For this review, take the finished solid that the model builds, in its own axes (mm). Coordinates: 2 decimals unless noted, no trailing zeros. Loops run counter-clockwise (first coordinate to the right, second up) from the corner with the lowest first, then second, coordinate; pieces in that order, holes last. Notation, with made-up numbers: (-30.75, 51) - (-21.75, 51) arc R32 cw to (-21.75, 77) - close; hole circle Ø7 at (51, 20). An arc over 180 degrees is marked (long way). One line per item, written item: value. Start each with the question number.
1. Take a section at B-B, the plane x = -1.7. State the section outline as (y, z) points.
2. To check wall thickness, follow line 1 (Z direction, x = -0.35, y = 0); line 2 (Z direction, x = 0.35, y = 3.75); line 3 (Y direction, x = -0.55, z = 1.5). State the ranges of each line that lie inside material, in increasing order. Write a range as from..to.
3. The part is to be moulded in two halves that separate along Y. For faces 1 (the face through (0, 0, -7)), 2 (the face through (1.893, -7.184, -0.158)), 3 (the face through (0.02, -3.54, -2.71)), say which applies: released by +Y, released by -Y, zero draft, split by the parting line, or undercut.
4. Take a section at A-A, the plane x = 0.45. State the section outline as (y, z) points.
5. Insertion check: pin 1 (6 mm diameter, centred on y = 0, z = 1.5, fed in from +X); pin 2 (5 mm diameter, centred on y = 1, z = -3, fed in from -X); pin 3 (2 mm diameter, centred on x = 1, z = 4, fed in from -Y); pin 4 (8 mm diameter, centred on y = 0, z = 0, fed in from -X). Each pin has a flat end and moves straight along its axis. Give the tip position at first contact, or say it passes through.
Autodesk Inventor part; units mm, degrees
ref_plane "nt_XY" through (0, 0, 0) normal (1, 0, 0) x (0, 0, -1)
ref_plane "nt_YZ" through (0, 0, 0) normal (0, 0, -1) x (0, 1, 0)
ref_plane "nt_ZX" through (0, 0, 0) normal (0, 1, 0) x (1, 0, 0)
sketch "B" plane through (0, 0, 0) normal (1, 0, 0) x (0, 1, 0)
  line L0 (-4.0415, 7) -> (-8.0829, 0)
  line L1 (-8.0829, 0) -> (-4.0415, -7)
  line L2 (-4.0415, -7) -> (4.0415, -7)
  line L3 (4.0415, -7) -> (8.0829, 0)
  line L4 (8.0829, 0) -> (4.0415, 7)
  line L5 (4.0415, 7) -> (-4.0415, 7)
extrude "Extrusion1" add sketch "B" along normal mid plane 4
sketch "Sketch_2" plane through (0, 0, 0) normal (0, 0, 1) x (1, 0, 0)
  line L0 (2, 0) -> (-2, 0)
  line L1 (-2, 0) -> (-2, 5)
  line L2 (-2, 5) -> (-1.4585, 4.4585)
  line L3 (-1.4585, 4.4585) -> (1.4585, 4.4585)
  line L4 (1.4585, 4.4585) -> (2, 5)
  line L5 (2, 5) -> (2, 0)
  line L6 (2, 0) -> (-2, 0)
revolve "Revolution1" cut sketch "Sketch_2" angle 360 about axis through (2, 0, 0) along (1, 0, 0)
thread "Thread1"
sketch "Sketch_3" plane through (0, 0, 0) normal (0, 0, 1) x (1, 0, 0)
  line L0 (50, 0) -> (-50, 0)
  line L1 (-7, 1) -> (-2, 1)
  line L2 (-2, 1) -> (-2, 7)
  line L3 (-2, 7) -> (0, 10.4641)
  line L4 (0, 10.4641) -> (2, 7)
  line L5 (2, 7) -> (2, 1)
  line L6 (2, 1) -> (7, 1)
  line L7 (7, 1) -> (7, 17)
  line L8 (7, 17) -> (-7, 17)
  line L9 (-7, 17) -> (-7, 1)
revolve "Revolution2" cut sketch "Sketch_3" angle 360 about axis through (50, 0, 0) along (1, 0, 0)
ref_plane "nt_XY" through (0, 0, 0) normal (1, 0, 0) x (0, 0, -1)
ref_plane "nt_YZ" through (0, 0, 0) normal (0, 0, -1) x (0, 1, 0)
ref_plane "nt_ZX" through (0, 0, 0) normal (0, 1, 0) x (1, 0, 0)
ref_plane "ntj_XY" through (2, 0, 0) normal (1, 0, 0) x (0, 0, -1)
ref_plane "ntj_YZ" through (2, 0, 0) normal (0, 0, -1) x (0, 1, 0)
ref_plane "ntj_ZX" through (2, 0, 0) normal (0, 1, 0) x (1, 0, 0)
properties part number "SNJ-016C"
Solutions:
1. outline: (-7.44, -1.12) - (-4.69, -5.88) arc R7.52 ccw to (-2.75, -7) - (2.75, -7) arc R7.52 ccw to (4.69, -5.88) - (7.44, -1.12) arc R7.52 ccw to (7.44, 1.12) - (4.69, 5.88) arc R7.52 ccw to (2.75, 7) - (-2.75, 7) arc R7.52 ccw to (-4.69, 5.88) - (-7.44, 1.12) arc R7.52 ccw to start; hole circle Ø9.4 at (0, 0)
2. line 1: -7..-4.46, 4.46..7
2. line 2: -7..-2.41, 2.41..7
2. line 3: -7.22..-4.2, 4.2..7.22
3. face 1: zero draft
3. face 2: released by -Y
3. face 3: undercut
4. outline: (-8.08, 0) - (-4.04, -7) - (4.04, -7) - (8.08, 0) - (4.04, 7) - (-4.04, 7) - close; hole circle Ø8.92 at (0, 0)
5. pin 1: x = 1.5
5. pin 2: x = -2
5. pin 3: y = -6.35
5. pin 4: through
